from build123d import *

# Parameters (mm, degrees)
F1_DEPTH = 5
F2_W     = 120
F2_H     = 2.8
F3_DEPTH = 10
F4_R     = 2.005
F5_DEPTH = 2.801
F7_DEPTH = 2.801


with BuildPart() as f1:
    # F0 (on Front) → F1 (new body)
    with BuildSketch(Plane.XZ):
        with BuildLine():
            Line((-29.8, -13.9), (29.8, -13.9))
            ThreePointArc((29.8, -13.9), (43.7, 0), (29.8, 13.9))
            Line((29.8, 13.9), (-29.8, 13.9))
            ThreePointArc((-29.8, 13.9), (-43.7, 0), (-29.8, -13.9))
        make_face()
        with BuildLine():
            ThreePointArc((29.8, 11.1), (40.9, 0), (29.8, -11.1))
            Line((29.8, -11.1), (-29.8, -11.1))
            ThreePointArc((-29.8, -11.1), (-40.9, 0), (-29.8, 11.1))
            Line((-29.8, 11.1), (29.8, 11.1))
        make_face(mode=Mode.SUBTRACT)
    extrude(amount=F1_DEPTH)

    # F2 (on face) → F3 (join)
    with BuildSketch(Plane.XZ.offset(5)):
        with Locations((0, -12.5)):
            Rectangle(F2_W, F2_H)
    extrude(amount=-F3_DEPTH)

    # F4 (on face) → F5 (cut, through all)
    with BuildSketch(Plane.XY.offset(-11.1)):
        with Locations((50, 0)):
            Circle(F4_R)
        with Locations((-50, 0)):
            Circle(F4_R)
    extrude(amount=-F5_DEPTH, mode=Mode.SUBTRACT)

    # F6 (on face) → F7 (cut, through all)
    with BuildSketch(Plane.XY.offset(-11.1)):
        with BuildLine():
            ThreePointArc((-50, -5), (-55, 0), (-50, 5))
            Line((-50, 5), (-60, 5))
            Line((-60, 5), (-60, -5))
            Line((-60, -5), (-50, -5))
        make_face()
        with BuildLine():
            Line((60, 5), (50, 5))
            ThreePointArc((50, 5), (55, 0), (50, -5))
            Line((50, -5), (60, -5))
            Line((60, -5), (60, 5))
        make_face()
    extrude(amount=-F7_DEPTH, mode=Mode.SUBTRACT)


solid = f1.part
Check sheet for the modelled part. Datum: model origin and axes. Units: mm. A direction names the side the tool comes from. Round coordinates to 2 decimals unless told otherwise and drop trailing zeros. Write each loop counter-clockwise with the first axis right and the second up, starting at its lowest first coordinate (ties: lowest second). Pieces come first, ordered by that corner, then holes. Notation, with made-up numbers: (13, 69) -> (37, 69) arc R24 ccw to (37, 95) -> close; hole circle Ø3 at (86.5, 5.25). An arc over 180 degrees is marked (long way). Answer as CSV lines item,"result". Start each with the question number.
1) Go/stop test with flat-tipped pins: P1, Ø8, axis at x = -26, z = -10, coming from the -Y side; P2, Ø3.5, axis at x = 50, y = 0, coming from the -Z side (3 decimals); P3, Ø5, axis at y = 0, z = 2, coming from the +X side. Record where each tip stops, or that it passes through.
2) Material ranges on line 1 (Z direction, x = -1.5, y = -1.75); line 2 (Z direction, x = -42, y = 3.5); line 3 (X direction, y = -0.25, z = -7.5), recorded low to high. Write a range as from..to.
3) Section check A-A on x = 26.5. Enter the section's corners in (y, z), and give its area (3 significant figures).
4) Section check B-B on z = 0. Enter the section's corners in (x, y).
5) Tool access check on faces 1 (the cylindrical face through (-40.9, -2.5, -0.2)), 2 (the flat face through (0, 0, 12)), 3 (the flat face through (0, -2, 13.9)). Record the directions out of +Z, -Z, +X, -X, +Y, -Y that give a thin tool (end or side, any length) a straight path to the whole face; none if there is none.
6) Release check for a two-part mould opening along Z. For faces 4 (the flat face through (0, -2, 11.1)), 5 (the cylindrical face through (-55, 0, -12)), 6 (the cylindrical face through (-42.902, -2.465, 4.641)), 7 (the flat face through (-1, 0, -13.9)) record: pulls with the +Z half, pulls with the -Z half, needs draft (parallel to the pull), parting line crosses it, or undercut.
Found:
1,P1,"stops at y = -5"
1,P2,"passes through"
1,P3,"stops at x = 43.7"
2,line 1,"z = -13.9..-11.1, 11.1..13.9"
2,line 2,"z = -13.9..-11.1"
2,line 3,"x = -41.5..-37.98, 37.98..41.5"
3,outline,"(-5, -13.9) -> (5, -13.9) -> (5, -11.1) -> (-5, -11.1) -> close; (-5, 11.1) -> (0, 11.1) -> (0, 13.9) -> (-5, 13.9) -> close"
3,area,"42.0 mm^2"
4,outline,"(-43.7, -5) -> (-40.9, -5) -> (-40.9, 0) -> (-43.7, 0) -> close; (40.9, -5) -> (43.7, -5) -> (43.7, 0) -> (40.9, 0) -> close"
5,face 1,"+Y, -Y"
5,face 2,"+Z, +X, -X, +Y"
5,face 3,"+Z, +X, -X, +Y, -Y"
6,face 4,"undercut"
6,face 5,"needs draft"
6,face 6,"undercut"
6,face 7,"pulls with the -Z half"
